The model under review builds one solid part; all positions refer to its coordinate system, in mm. Face numbers are marked on the shaded views. A direction names the side the tool comes from. Coordinates: 2 decimals unless noted, no trailing zeros. Write each loop counter-clockwise with the first axis right and the second up, starting at its lowest first coordinate (ties: lowest second). Pieces come first, ordered by that corner, then holes. Notation, with made-up numbers: M 43.25,15.25 L 66.25,15.25 A22 cw 66.25,30.25 Z; hole C 62,83 d8. An arc over 180 degrees is marked long. Answer as a JSON object with one key per item and string values.
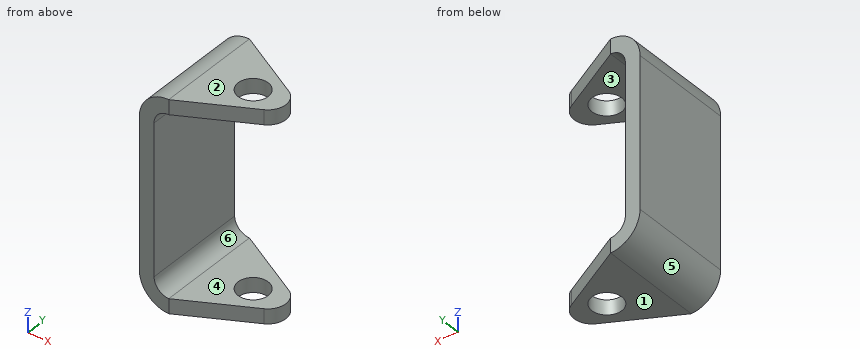
Solid Edge part; units mm, degrees
sketch "Sketch1" plane through (0, 0, 0) normal (0, 1, 0) x (-1, 0, 0)
  line L0 (0, 25.5) -> (0, 0)
  line L1 (0, 0) -> (-5, 0)
  line L2 (-5, 0) -> (-5, 25.5)
  arc A0 (-10, 30.5) -> (-5, 25.5) centre (-10, 25.5) cw
  line L3 (-50, 30.5) -> (-10, 30.5)
  line L4 (-50, 35.5) -> (-50, 30.5)
  line L5 (-10, 35.5) -> (-50, 35.5)
  arc A1 (-10, 35.5) -> (0, 25.5) centre (-10, 25.5) cw
extrude "Protrusion1" add sketch "Sketch1" along normal mid plane 35
hole "Hole_1" at (25, 0, 35.5) direction (0, 0, -1) diameter 10.2 end up to next
sketch "Sketch2" plane through (40, 0, 35.5) normal (0, 0, 1) x (0, 1, 0)
  line L0 (-17.5, 30) -> (-5.3902, 7.1441)
  arc A0 (-5.3902, 7.1441) -> (5.3902, 7.1441) centre (0, 10) ccw
  line L1 (17.5, 30) -> (5.3902, 7.1441)
extrude "Cutout1" cut sketch "Sketch2" against normal up to next material side at (21.4514, -11.4893, 35.5)
mirror "Mirror1" about plane through (5, 0, 0) normal (0, 0, -1) of "Protrusion1", "Cutout1", "Hole_1"
(1) Add section B-B on x = 21.5. Give the boundary of the cut face in (y, z), and give its area (3 significant figures).
Results list:
{"outline": "M -11.41,-35.5 L -3.71,-35.5 L -3.71,-30.5 L -11.41,-30.5 Z; M -11.41,30.5 L -3.71,30.5 L -3.71,35.5 L -11.41,35.5 Z; M 3.71,-35.5 L 11.41,-35.5 L 11.41,-30.5 L 3.71,-30.5 Z; M 3.71,30.5 L 11.41,30.5 L 11.41,35.5 L 3.71,35.5 Z", "area": "154 mm²"}
(2) Add section D-D on y = -12. Give the boundary of the cut face in (x, z), and give its area (3 significant figures).
Results list:
{"outline": "M 0,-25.5 A10 ccw 10,-35.5 L 20.38,-35.5 L 20.38,-30.5 L 10,-30.5 A5 cw 5,-25.5 L 5,25.5 A5 cw 10,30.5 L 20.38,30.5 L 20.38,35.5 L 10,35.5 A10 ccw 0,25.5 Z", "area": "477 mm²"}
(3) Add section A-A on y = 0. Give the boundary of the cut face in (x, z).
Results list:
{"outline": "M 0,-25.5 A10 ccw 10,-35.5 L 19.9,-35.5 L 19.9,-30.5 L 10,-30.5 A5 cw 5,-25.5 L 5,25.5 A5 cw 10,30.5 L 19.9,30.5 L 19.9,35.5 L 10,35.5 A10 ccw 0,25.5 Z; M 30.1,-35.5 L 36.1,-35.5 L 36.1,-30.5 L 30.1,-30.5 Z; M 30.1,30.5 L 36.1,30.5 L 36.1,35.5 L 30.1,35.5 Z"}
(4) Wall thickness on line 1 along Z through (x, y) = (13, 13.5); line 2 along X through (y, z) = (0, -3.5); line 3 along X through (y, z) = (0, -31): over which ranges is each line inside the solid? List them lowest first. Write a range as from..to.
Results list:
{"line 1": "-35.5..-30.5, 30.5..35.5", "line 2": "0..5", "line 3": "1.65..19.9, 30.1..36.1"}
(5) For the marked faces 5 and 6, list the 3-axis set-ups (+Z, -Z, +X, -X, +Y, -Y) from which the entire face can be reached by the end or side of a thin tool; tool diameter is ignored.
Results list:
{"face 5": "-Z, -X, +Y, -Y", "face 6": "+X, +Y, -Y"}
(6) Add section C-C on x = 16. Give the boundary of the cut face in (y, z).
Results list:
{"outline": "M -14.32,-35.5 L 14.32,-35.5 L 14.32,-30.5 L -14.32,-30.5 Z; M -14.32,30.5 L 14.32,30.5 L 14.32,35.5 L -14.32,35.5 Z"}
(7) Draft analysis for pull direction Z (two halves, no side actions). For the marked faces 1, 2, 3 and 4, state which applies: released by +Z, released by -Z, zero draft, split by the parting line, or undercut.
Results list:
{"face 1": "released by -Z", "face 2": "released by +Z", "face 3": "undercut", "face 4": "undercut"}
(8) For pin 1 Ø6 at (y, z) = (13.5, -1) entering from +X; pin 2 Ø1 at (x, y) = (7.5, -5.5) entering from +Z, all flat-tipped, find the tip position at first contact; note any pin that passes through.
Results list:
{"pin 1": "x = 5", "pin 2": "z = 35.3"}
